Geometry: final body of the model. Coordinates: model frame, mm. A direction names the side the tool comes from. Give positions to 0.01 mm unless a question says otherwise; leave off trailing zeros. Write each loop counter-clockwise with the first axis right and the second up, starting at its lowest first coordinate (ties: lowest second). Pieces come first, ordered by that corner, then holes. Notation, with made-up numbers: (76, 62.25) -> (82, 62.25) arc R17 cw to (82, 66.25) -> close; hole circle Ø1 at (82, -36). An arc over 180 degrees is marked (long way). Answer as a JSON object with one key per item and string values.
from build123d import *

# Parameters (mm, degrees)
BOSS_EXTRUDE1_DEPTH      = 26.924
BOSS_EXTRUDE1_DEPTH_BACK = 26.924
SKETCH1_R                = 8
BOSS_EXTRUDE2_DEPTH      = 26.924
BOSS_EXTRUDE2_DEPTH_BACK = 26.924
SKETCH2_R                = 8


with BuildPart() as part:
    # Sketch1 → Boss-Extrude1 (new, two sides: drawn at the far end of the back side and taken through both)
    with BuildSketch(Plane(origin=(0, 0, 0), x_dir=(1, 0, 0), z_dir=(0, 1, 0)).offset(-BOSS_EXTRUDE1_DEPTH_BACK)):
        with Locations(Location((0, 0, 0), (0, 0, 270))):
            Circle(SKETCH1_R)
    extrude(amount=BOSS_EXTRUDE1_DEPTH + BOSS_EXTRUDE1_DEPTH_BACK)

    # Sketch2 → Boss-Extrude2 (add, two sides: drawn at the far end of the back side and taken through both)
    with BuildSketch(Plane.XY.offset(-BOSS_EXTRUDE2_DEPTH_BACK)):
        Circle(SKETCH2_R)
    extrude(amount=BOSS_EXTRUDE2_DEPTH + BOSS_EXTRUDE2_DEPTH_BACK)


solid = part.part
Q1. Cut plane A-A (x = 0). Return the cut outline in (y, z), and give its area (3 significant figures).
Values:
{"outline": "(-26.92, -8) -> (-8, -8) -> (-8, -26.92) -> (8, -26.92) -> (8, -8) -> (26.92, -8) -> (26.92, 8) -> (8, 8) -> (8, 26.92) -> (-8, 26.92) -> (-8, 8) -> (-26.92, 8) -> close", "area": "1,470 mm²"}
Q2. First-contact query: P1, Ø3, axis at y = -6, z = -13.5, coming from the -X side; P2, Ø5, axis at y = 13.5, z = -12.5, coming from the +X side; P3, Ø5, axis at x = 1, y = 11.5, coming from the +Z side; P4, Ø4, axis at x = -3, z = -11.5, coming from the +Y side. Flat tips, straight axial feed; report the tip coordinate or a pass-through.
Values:
{"P1": "x = -6.61", "P2": "through", "P3": "z = 8", "P4": "y = 7.94"}
Q3. Set-up query: faces 1 (the flat face through (0, 26.924, 0)), 2 (the cylindrical face through (0, 16, -8)), 3 (the cylindrical face through (7.39, -3.06, -16.64)), 4 (the cylindrical face through (2.4, -16.64, 7.63)), 5 (the cylindrical face through (7.39, -3.06, 16.27)). Return all of +Z, -Z, +X, -X, +Y, -Y with unobstructed straight access to the full face (end or side cutting, diameter ignored); none if empty.
Values:
{"face 1": "+Z, -Z, +X, -X, +Y", "face 2": "+Y", "face 3": "-Z", "face 4": "-Y", "face 5": "+Z"}
Q4. Cut plane D-D (z = 15). Return the cut outline in (x, y).
Values:
{"outline": "circle Ø16 at (0, 0)"}
Q5. Cut plane C-C (z = 4.5). Return the cut outline in (x, y), and give its area (3 significant figures).
Values:
{"outline": "(-6.61, -26.92) -> (6.61, -26.92) -> (6.61, -4.5) arc R8 ccw to (6.61, 4.5) -> (6.61, 26.92) -> (-6.61, 26.92) -> (-6.61, 4.5) arc R8 ccw to (-6.61, -4.5) -> close", "area": "729 mm²"}
Q6. Cut plane B-B (y = -5). Return the cut outline in (x, z) (3 decimals), and give its area (3 significant figures).
Values:
{"outline": "(-6.245, -26.924) -> (6.245, -26.924) -> (6.245, -5) arc R8 ccw to (6.245, 5) -> (6.245, 26.924) -> (-6.245, 26.924) -> (-6.245, 5) arc R8 ccw to (-6.245, -5) -> close", "area": "697 mm²"}
Q7. Material intervals for L1, parallel to Y at x = 0, z = 11.5; L2, parallel to Z at x = 4, y = 13; L3, parallel to X at y = 4.5, z = 14, sorted ascending. Write a range as from..to.
Values:
{"L1": "-8..8", "L2": "-6.93..6.93", "L3": "-6.61..6.61"}
